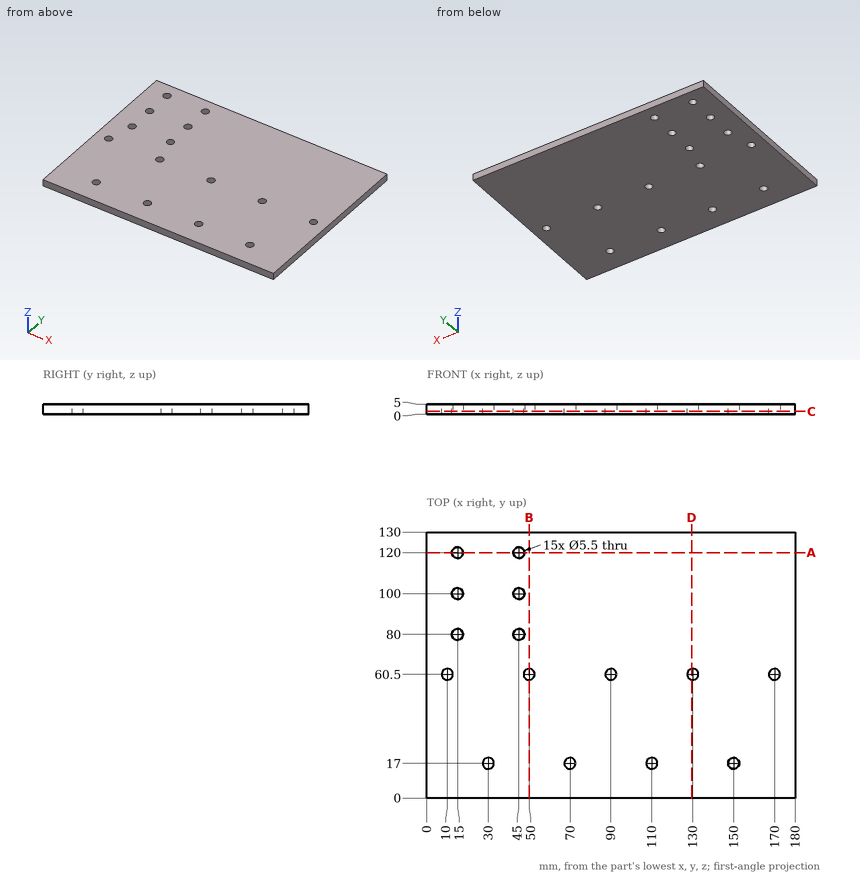
Answer from the drawing. Dimensions are ordinates in mm from the lowest x, y and z of the part. Round coordinates to 2 decimals unless told otherwise and drop trailing zeros. Order: outer loops, then holes, each group sorted by start corner. A loop starts at its lowest first (then second) coordinate and runs counter-clockwise, first axis right, second up.
1) The part is cut by section C-C on z = 1.45. Give the number of separate pieces and of enclosed holes in the cut face, plus the area to 3 significant figures.
2) The part is cut by section A-A on y = 120. Write down the section's boundary in (x, z).
3) The part is cut by section D-D on x = 129.5. Write down the section's boundary in (y, z).
4) Straight lines are drawn through the part: L1, parallel to Y at x = 45, z = 3.5; L2, parallel to X at y = 120, z = 2.6; L3, parallel to Y at x = 130, z = 2.9. For each, find the intervals that lie inside material, in ascending order.
5) The part is cut by section B-B on x = 50. Write down the section's boundary in (y, z), plus the area to 4 significant figures.
Resolved:
1. separate pieces: 1
1. enclosed holes: 15
1. area: 23,000 mm2
2. outline: (0, 0) - (12.25, 0) - (12.25, 5) - (0, 5) - close; (17.75, 0) - (42.25, 0) - (42.25, 5) - (17.75, 5) - close; (47.75, 0) - (180, 0) - (180, 5) - (47.75, 5) - close
3. outline: (0, 0) - (57.8, 0) - (57.8, 5) - (0, 5) - close; (63.2, 0) - (130, 0) - (130, 5) - (63.2, 5) - close
4. L1: y = 0 to 77.25, 82.75 to 97.25, 102.75 to 117.25, 122.75 to 130
4. L2: x = 0 to 12.25, 17.75 to 42.25, 47.75 to 180
4. L3: y = 0 to 57.75, 63.25 to 130
5. outline: (0, 0) - (57.75, 0) - (57.75, 5) - (0, 5) - close; (63.25, 0) - (130, 0) - (130, 5) - (63.25, 5) - close
5. area: 622.5 mm2
